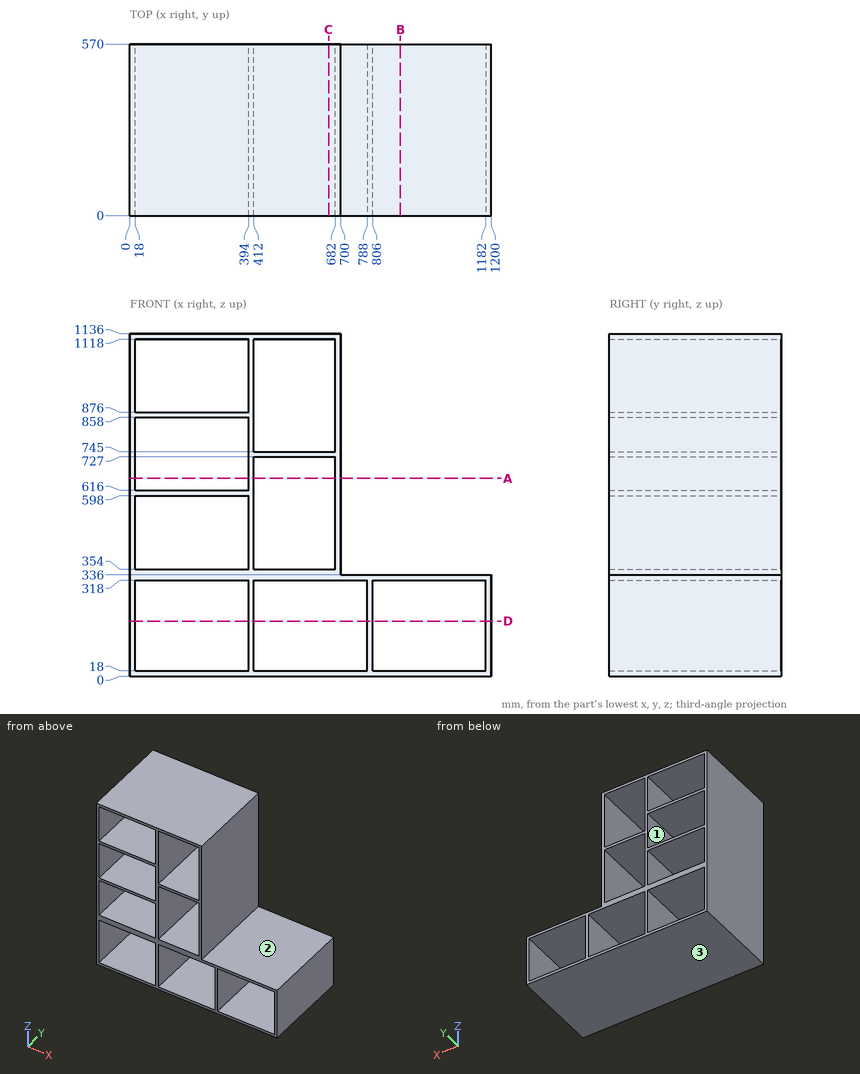
Could you check a few things on this drawing? It's one solid part, dimensions in mm from its lowest x, y, z. Give positions to 0.01 mm unless a question says otherwise; leave off trailing zeros. Order: outer loops, then holes, each group sorted by start corner. A loop starts at its lowest first (then second) coordinate and runs counter-clockwise, first axis right, second up. Notation, with made-up numbers: (-25.75, -8.75) - (-2.75, -8.75) arc R21 ccw to (-2.75, 14.25) - close; hole circle Ø8 at (-35.5, 0.5). An arc over 180 degrees is marked (long way). Answer as a JSON object with one key per item and string values. Group by question number.
Item 1: If we section it at B-B on x = 897.5: Please give me the cut outline in (y, z).
Item 2: For P1, Ø3, axis at y = 455, z = 839, coming from the -X side; P2, Ø1.5, axis at y = 191, z = 959.5, coming from the +X side; P3, Ø10, axis at x = 731.5, y = 130.5, coming from the +Z side, each with a flat end and sliding along its axis, tell me the tip position at first contact or that it passes through.
Item 3: If we mould it in two halves opening along Z, with no side actions, what happens to the marked faces 1, 2 and 3? For each: pulls with the +Z half, pulls with the -Z half, needs draft (parallel to the pull), parting line crosses it, or undercut.
Item 4: Please list where these lines run through material, in increasing order: probe 1 along X at (y, z) = (123, 1051); probe 2 along Z at (x, y) = (569, 65); probe 3 along Z at (x, y) = (185.5, 208.5).
Item 5: If we section it at D-D on z = 182.5: Please give me the cut outline in (x, y).
Item 6: If we section it at A-A on z = 656: Please give me the cut outline in (x, y).
Item 7: If we section it at C-C on x = 659.5: Please give me the cut outline in (y, z).
Result set:
{
 "1": {"outline": "(0, 0) - (570, 0) - (570, 18) - (0, 18) - close; (0, 318) - (570, 318) - (570, 336) - (0, 336) - close"},
 "2": {"P1": "x = 0", "P2": "x = 700", "P3": "z = 336"},
 "3": {"face 1": "undercut", "face 2": "pulls with the +Z half", "face 3": "pulls with the -Z half"},
 "4": {"probe 1": "0 to 18, 394 to 412, 682 to 700", "probe 2": "0 to 18, 318 to 354, 727 to 745, 1118 to 1136", "probe 3": "0 to 18, 318 to 354, 598 to 616, 858 to 876, 1118 to 1136"},
 "5": {"outline": "(0, 0) - (18, 0) - (18, 570) - (0, 570) - close; (394, 0) - (412, 0) - (412, 570) - (394, 570) - close; (788, 0) - (806, 0) - (806, 570) - (788, 570) - close; (1182, 0) - (1200, 0) - (1200, 570) - (1182, 570) - close"},
 "6": {"outline": "(0, 0) - (18, 0) - (18, 570) - (0, 570) - close; (394, 0) - (412, 0) - (412, 570) - (394, 570) - close; (682, 0) - (700, 0) - (700, 570) - (682, 570) - close"},
 "7": {"outline": "(0, 0) - (570, 0) - (570, 18) - (0, 18) - close; (0, 318) - (570, 318) - (570, 354) - (0, 354) - close; (0, 727) - (570, 727) - (570, 745) - (0, 745) - close; (0, 1118) - (570, 1118) - (570, 1136) - (0, 1136) - close"}
}
